Verification items for this drawing (mm, ordinates from the low corner). A direction names the side the tool comes from. Coordinates: 2 decimals unless noted, no trailing zeros. Loops run counter-clockwise (first coordinate to the right, second up) from the corner with the lowest first, then second, coordinate; pieces in that order, holes last. Notation, with made-up numbers: M -5,62.25 L 43,62.25 A22 ccw 43,90.25 Z; hole C 62,10 d1. An arc over 180 degrees is marked long. Use CSV: the item, a comma, the result in double quotes.
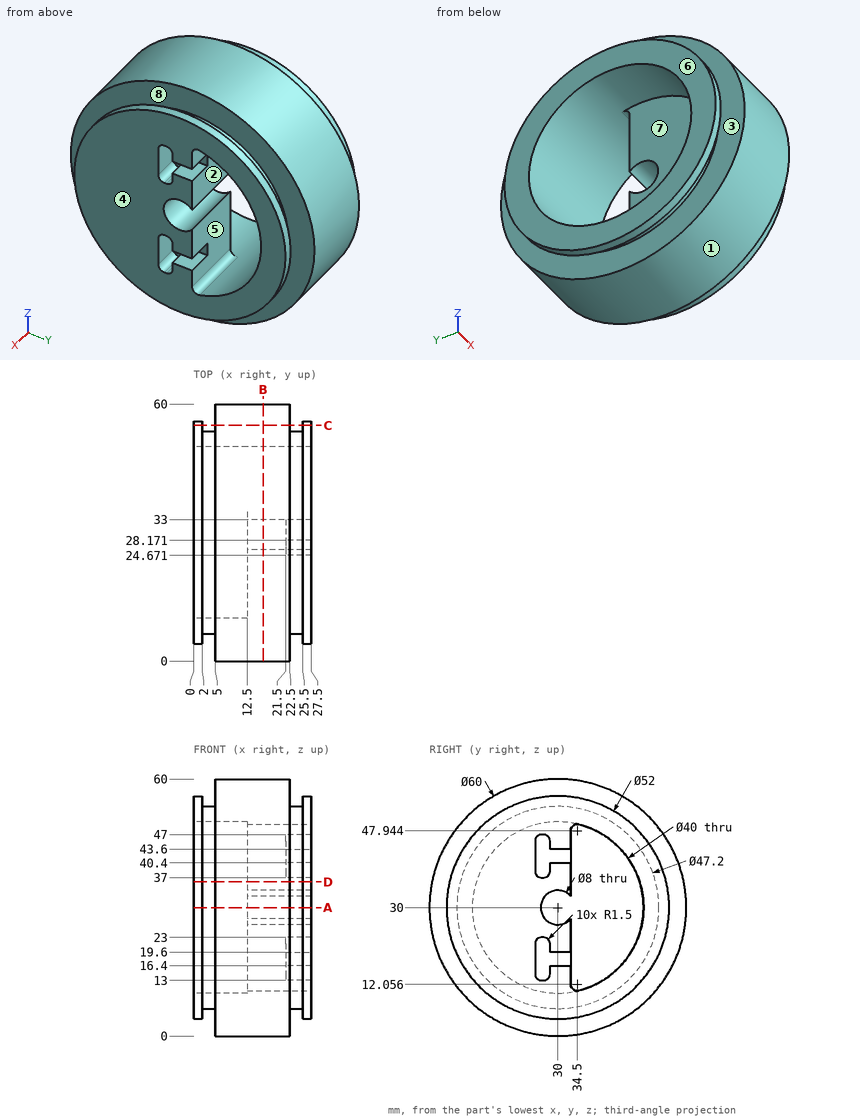
1. Section check D-D, the plane z = 36. Record the cut outline in (x, y) (1 decimal), plus the area to 3 significant figures.
The answers:
outline,"M 0,4.7 L 2,4.7 L 2,7.2 L 5,7.2 L 5,0.6 L 22.5,0.6 L 22.5,7.2 L 25.5,7.2 L 25.5,4.7 L 27.5,4.7 L 27.5,33 L 12.5,33 L 12.5,10.9 L 0,10.9 Z; M 0,49.1 L 27.5,49.1 L 27.5,55.3 L 25.5,55.3 L 25.5,52.8 L 22.5,52.8 L 22.5,59.4 L 5,59.4 L 5,52.8 L 2,52.8 L 2,55.3 L 0,55.3 Z"
area,"787 mm^2"
2. Section check A-A, the plane z = 30. Record the cut outline in (x, y).
The answers:
outline,"M 0,4 L 2,4 L 2,6.4 L 5,6.4 L 5,0 L 22.5,0 L 22.5,6.4 L 25.5,6.4 L 25.5,4 L 27.5,4 L 27.5,26 L 12.5,26 L 12.5,10 L 0,10 Z; M 0,50 L 27.5,50 L 27.5,56 L 25.5,56 L 25.5,53.6 L 22.5,53.6 L 22.5,60 L 5,60 L 5,53.6 L 2,53.6 L 2,56 L 0,56 Z"
3. Set-up check for the marked faces 4, 5, 6, 7 and 8: record each of +Z, -Z, +X, -X, +Y, -Y from which the full face is reachable in a straight line by a thin tool's end or side.
The answers:
face 4,"+Z, -Z, +X, +Y, -Y"
face 5,"+X, -X"
face 6,"+Z, -Z, -X, +Y, -Y"
face 7,"-X"
face 8,"none"
4. Gauge pin test, flat ends, axial feed: P1, Ø12, axis at x = 15.5, y = 27, coming from the +Z side; P2, Ø7.5, axis at x = 23, z = 42, coming from the +Y side; P3, Ø1.5, axis at x = 24, z = 39.5, coming from the -Y side; P4, Ø5, axis at y = 30, z = 30, coming from the +X side. Record the tip position at first contact, or that the pin passes through.
The answers:
P1,"z = 60"
P2,"y = 58.83"
P3,"y = 8.08"
P4,"through"
5. Section check B-B, the plane x = 16.25. Record the cut outline in (y, z) (1 decimal).
The answers:
outline,"C 30,30 d60; hole M 33,12.1 A1.5 ccw 34.9,10.6 A20 ccw 34.9,49.4 A1.5 ccw 33,47.9 L 33,32.6 A4 ccw long 33,27.4 Z"
6. Release check for a two-part mould opening along Y. For the marked faces 1, 2 and 3 record: +Y half, -Y half, draft (parallel to the pull), parting line (faces both ways), or undercut.
The answers:
face 1,"parting line"
face 2,"undercut"
face 3,"draft"
7. Section check C-C, the plane y = 55. Record the cut outline in (x, z).
The answers:
outline,"M 0,22.86 L 2,22.86 L 2,37.14 L 0,37.14 Z; M 5,13.42 L 22.5,13.42 L 22.5,46.58 L 5,46.58 Z; M 25.5,22.86 L 27.5,22.86 L 27.5,37.14 L 25.5,37.14 Z"
8. Thickness scan on line 1 (Y direction, x = 16, z = 33.5) (1 decimal); line 2 (Z direction, x = 19.5, y = 30); line 3 (Z direction, x = 6.25, y = 30). Record the ranges inside material, lowest first. Write a range as [from, to].
The answers:
line 1,"[0.2, 28.1], [31.9, 33], [49.7, 59.8]"
line 2,"[0, 26], [34, 60]"
line 3,"[0, 10], [50, 60]"
